Could you check a few things on this model? Use its own coordinates, in mm. Face numbers are marked on the shaded views. A direction names the side the tool comes from. Give positions to 0.01 mm unless a question says otherwise; leave off trailing zeros. Loops run counter-clockwise (first coordinate to the right, second up) from the corner with the lowest first, then second, coordinate; pieces in that order, holes last. Notation, with made-up numbers: M 25,74 L 31,74 A21 ccw 31,91 Z; hole C 50,14 d7. An arc over 180 degrees is marked long. Use CSV: the item, a comma, the result in double quotes.
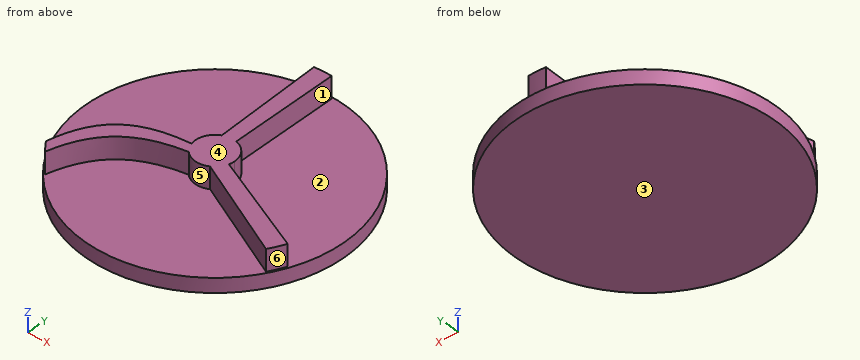
```python
from build123d import *

# Parameters (mm, degrees)
F1_DEPTH = 7.62
F2_R     = 45.72373
F3_DEPTH = 5.08


with BuildPart() as f1:
    # F0 (on Top) → F1 (new body)
    with BuildSketch(Plane.XY):
        with BuildLine():
            ThreePointArc((-3.120344, 6.258425), (-0.834145, 6.943244), (1.549203, 6.819414))
            Line((1.549203, 6.819414), (1.549203, 45.108627))
            ThreePointArc((1.549203, 45.108627), (-1.503064, 45.110188), (-4.548458, 44.905454))
            Line((-4.548458, 44.905454), (-3.120344, 6.258425))
        make_face()
        with BuildLine():
            ThreePointArc((-4.890711, -4.998538), (-6.047151, -3.512321), (-6.765095, -1.771418))
            add(Edge.make_bspline(
                [(-6.765095, -1.771418), (-25.271352, -2.981601), (-33.291422, -10.951445), (-36.469723, -26.592246)],
                knots=[0, 0, 0, 0, 38.709668, 38.709668, 38.709668, 38.709668], degree=3))
            ThreePointArc((-36.469723, -26.592246), (-35.071161, -28.411299), (-33.58196, -30.156927))
            add(Edge.make_bspline(
                [(-4.890711, -4.998538), (-20.500017, -7.315121), (-29.63965, -14.453498), (-33.58196, -30.156927)],
                knots=[0, 0, 0, 0, 38.159301, 38.159301, 38.159301, 38.159301], degree=3))
        make_face()
        with BuildLine():
            Line((41.473617, -17.80807), (6.700846, -2.000774))
            ThreePointArc((6.700846, -2.000774), (5.510265, -4.305974), (3.561225, -6.018481))
            Line((3.561225, -6.018481), (38.651442, -23.307816))
            ThreePointArc((38.651442, -23.307816), (40.156793, -20.606314), (41.473617, -17.80807))
        make_face()
        with BuildLine():
            ThreePointArc((6.700846, -2.000774), (6.919704, -1.011008), (6.993171, 0))
            ThreePointArc((6.993171, 0), (5.465267, 4.362946), (1.549203, 6.819414))
            ThreePointArc((1.549203, 6.819414), (-0.834145, 6.943244), (-3.120344, 6.258425))
            ThreePointArc((-3.120344, 6.258425), (-6.367894, 2.890391), (-6.765095, -1.771418))
            ThreePointArc((-6.765095, -1.771418), (-6.047151, -3.512321), (-4.890711, -4.998538))
            ThreePointArc((-4.890711, -4.998538), (-0.837827, -6.942801), (3.561225, -6.018481))
            ThreePointArc((3.561225, -6.018481), (5.510265, -4.305974), (6.700846, -2.000774))
        make_face()
    extrude(amount=F1_DEPTH)

    # F2 (on Top) → F3 (join)
    with BuildSketch(Plane.XY):
        Circle(F2_R)
    extrude(amount=-F3_DEPTH)


solid = f1.part
```
1. If we mould it in two halves opening along X, with no side actions, what happens to the marked faces 4, 5 and 6? For each: +X half, -X half, draft (parallel to the pull), parting line (faces both ways), or undercut.
Outcome:
face 4,"draft"
face 5,"undercut"
face 6,"+X half"
2. I'm going to push flat-ended pins straight in: pin 1 Ø5 at (x, y) = (27.5, 17) entering from +Z; pin 2 Ø6 at (x, z) = (-13.5, -1) entering from -Y; pin 3 Ø2.5 at (y, z) = (33, 3) entering from +X. Where does each tip first touch, or does it pass through?
Outcome:
pin 1,"z = 0"
pin 2,"y = -44.5"
pin 3,"x = 1.55"
3. Please list where these lines run through material, in increasing order: line 1 (Z direction, x = 0.5, y = -17); line 2 (X direction, y = -27, z = 1.5); line 3 (Y direction, x = -34.5, z = -0.5).
Outcome:
line 1,"-5.08 to 0"
line 2,"-36.17 to -32.68"
line 3,"-30.01 to 30.01"
4. Which directions (+Z, -Z, +X, -X, +Y, -Y) give clear straight access to the entire face, cutting with the end or side of a thin tool? Please do the marked faces 1, 2 and 3.
Outcome:
face 1,"+Z, +X, +Y"
face 2,"+Z"
face 3,"-Z, +X, -X, +Y, -Y"
5. I want a section at B-B, the plane y = 18. List the corners of the cut face in (x, z) for me.
Outcome:
outline,"M -42.03,-5.08 L 42.03,-5.08 L 42.03,0 L 1.55,0 L 1.55,7.62 L -3.55,7.62 L -3.55,0 L -42.03,0 Z"
6. I want a section at C-C, the plane z = -2.5. List the corners of the cut face in (x, y) for me.
Outcome:
outline,"C 0,0 d91.45"
7. I want a section at D-D, the plane y = -36.5. List the corners of the cut face in (x, z) for me.
Outcome:
outline,"M -27.54,-5.08 L 27.54,-5.08 L 27.54,0 L -27.54,0 Z"
8. I want a section at A-A, the plane x = 0. List the corners of the cut face in (y, z) for me.
Outcome:
outline,"M -45.72,-5.08 L 45.72,-5.08 L 45.72,0 L 45.14,0 L 45.14,7.62 L -6.99,7.62 L -6.99,0 L -45.72,0 Z"
